from build123d import *

# Parameters (mm, degrees)
BOSS_EXTRUDE1_DEPTH = 11
SKETCH2_R           = 0.5
CUT_EXTRUDE1_DEPTH  = 39.49675311
SKETCH3_W           = 9
SKETCH3_H           = 20
BOSS_EXTRUDE2_DEPTH = 0.5
SKETCH5_R           = 1.25
SKETCH5_R_2         = 2
BOSS_EXTRUDE3_DEPTH = 0.5
FILLET2_R           = 0.5
FILLET3_R           = 0.5
FILLET4_R           = 0.5
FILLET5_R           = 0.5
FILLET6_R           = 0.5
FILLET7_R           = 0.5
CUT_EXTRUDE3_START  = -0.3
CUT_EXTRUDE3_DEPTH  = 0.3


with BuildPart() as part:
    # Sketch1 → Boss-Extrude1 (new body)
    with BuildSketch(Plane(origin=(0, 0, 0), x_dir=(0, 0, -1), z_dir=(1, 0, 0))):
        Polygon((0, 0), (0, 31), (20, 31), (20, 6), (14, 0), align=None)
    extrude(amount=BOSS_EXTRUDE1_DEPTH)

    # Sketch2 → Cut-Extrude1 (cut, through all)
    with BuildSketch(Plane(origin=(11, 0, 0), x_dir=(0, 0, -1), z_dir=(1, 0, 0))):
        with Locations((3, 2.8)):
            Circle(SKETCH2_R)
        with Locations((3, 28.2)):
            Circle(SKETCH2_R)
    extrude(amount=-CUT_EXTRUDE1_DEPTH, mode=Mode.SUBTRACT)

    # Sketch3 → Boss-Extrude2 (add)
    with BuildSketch(Plane.XY):
        with Locations((5.5, 18)):
            Rectangle(SKETCH3_W, SKETCH3_H)
    extrude(amount=BOSS_EXTRUDE2_DEPTH)

    # Sketch5 → Boss-Extrude3 (add)
    with BuildSketch(Plane(origin=(0, 31, 0), x_dir=(1, 0, 0), z_dir=(0, 1, 0))):
        with Locations(Location((3.5, 3.5, 0), (0, 0, 90))):
            Circle(SKETCH5_R)
        with Locations(Location((7.5, 3.5, 0), (0, 0, 90))):
            Circle(SKETCH5_R)
        with Locations(Location((5.5, 15, 0), (0, 0, 90))):
            Circle(SKETCH5_R_2)
        with Locations(Location((5.5, 9, 0), (0, 0, 90))):
            Circle(SKETCH5_R_2)
    extrude(amount=BOSS_EXTRUDE3_DEPTH)

    # Fillet2
    fillet2_edges = [part.edges().sort_by_distance(p)[0] for p in [
        (3.5, 31.5, -2.25),
    ]]
    fillet(fillet2_edges, radius=FILLET2_R - 0.0001)  # a hair under: the kernel refuses the full size

    # Fillet3
    fillet3_edges = [part.edges().sort_by_distance(p)[0] for p in [
        (7.5, 31.5, -2.25),
    ]]
    fillet(fillet3_edges, radius=FILLET3_R - 0.0001)  # a hair under: the kernel refuses the full size

    # Fillet4
    fillet4_edges = [part.edges().sort_by_distance(p)[0] for p in [
        (5.5, 31, 0),
    ]]
    fillet(fillet4_edges, radius=FILLET4_R)

    # Fillet5
    fillet5_edges = [part.edges().sort_by_distance(p)[0] for p in [
        (5.5, 31, -20),
    ]]
    fillet(fillet5_edges, radius=FILLET5_R)

    # Fillet6
    fillet6_edges = [part.edges().sort_by_distance(p)[0] for p in [
        (5.5, 0, 0),
    ]]
    fillet(fillet6_edges, radius=FILLET6_R)

    # Fillet7
    fillet7_edges = [part.edges().sort_by_distance(p)[0] for p in [
        (5.5, 6, -20),
    ]]
    fillet(fillet7_edges, radius=FILLET7_R)

    # Sketch6 → Cut-Extrude3 (cut)
    with BuildSketch(Plane(origin=(0, 31.5, 0), x_dir=(1, 0, 0), z_dir=(0, 1, 0)).offset(CUT_EXTRUDE3_START)):
        with BuildLine():
            Line((6.786176444, 10.531584197), (3.6331206, 8.282531321))
            ThreePointArc((3.6331206, 8.282531321), (3.86671689, 7.84570962), (4.200507105, 7.479697985))
            Line((4.200507105, 7.479697985), (7.373069331, 9.701149971))
            ThreePointArc((7.373069331, 9.701149971), (7.13328311, 10.15429038), (6.786176444, 10.531584197))
        make_face()
        with BuildLine():
            Line((3.62088338, 14.315222133), (6.812710383, 16.508904056))
            ThreePointArc((6.812710383, 16.508904056), (7.143293876, 16.139993525), (7.373069331, 15.701149971))
            Line((7.373069331, 15.701149971), (4.200507105, 13.479697985))
            ThreePointArc((4.200507105, 13.479697985), (3.856706124, 13.860006475), (3.62088338, 14.315222133))
        make_face()
    extrude(amount=CUT_EXTRUDE3_DEPTH, mode=Mode.SUBTRACT)


solid = part.part
For this review, take the finished solid that the model builds, in its own axes (mm). A direction names the side the tool comes from. Round coordinates to 2 decimals unless told otherwise and drop trailing zeros. Write each loop counter-clockwise with the first axis right and the second up, starting at its lowest first coordinate (ties: lowest second). Pieces come first, ordered by that corner, then holes. Notation, with made-up numbers: (72, 72.25) - (110, 72.25) arc R19 cw to (110, 103.25) - close; hole circle Ø2 at (-30, -30.75). An arc over 180 degrees is marked (long way). Use a Markdown table: item, result.
Q1. Clearance check with flat-ended pins moving along their axes: pin 1 (0.6 mm diameter, centred on x = 6.5, z = 0.5, fed in from -Y); pin 2 (0.6 mm diameter, centred on x = 4, z = 0.5, fed in from +Y); pin 3 (3.5 mm diameter, centred on x = 4, z = -13, fed in from +Y). State where each tip first meets the part, or that it passes through.
Derived:
| item | result |
|---|---|
| pin 1 | stops at y = 8 |
| pin 2 | stops at y = 28 |
| pin 3 | stops at y = 31.5 |
Q2. Wall thickness on line 1 along Y through (x, z) = (6, -3); line 2 along Y through (x, z) = (4.5, -3); line 3 along Y through (x, z) = (6.5, -7): over which ranges is each line inside the solid? List them lowest first.
Derived:
| item | result |
|---|---|
| line 1 | y = 0 to 2.3, 3.3 to 27.7, 28.7 to 31 |
| line 2 | y = 0 to 2.3, 3.3 to 27.7, 28.7 to 31.34 |
| line 3 | y = 0 to 31 |
Q3. The part is to be moulded in two halves that separate along Y. For faces 3 (the flat face through (5.23, 31.35, -9.42)), 4 (the cylindrical face through (5.6, 2.5, -2.6)), 5 (the flat face through (5, 0, -7)), 6 (the flat face through (3.5, 31.5, -3.5)), say which applies: pulls with the +Y half, pulls with the -Y half, needs draft (parallel to the pull), parting line crosses it, or undercut.
Derived:
| item | result |
|---|---|
| face 3 | needs draft |
| face 4 | undercut |
| face 5 | pulls with the -Y half |
| face 6 | pulls with the +Y half |
Q4. We need section B-B (z = -11.75). Give the boundary of the cut face in (x, y), plus the area to 3 significant figures.
Derived:
| item | result |
|---|---|
| outline | (0, 0) - (11, 0) - (11, 31) - (0, 31) - close |
| area | 341 mm2 |
Q5. We need section A-A (x = 1.75). Give the boundary of the cut face in (y, z), plus the area to 3 significant figures.
Derived:
| item | result |
|---|---|
| outline | (0, -14) - (5.85, -19.85) arc R0.5 ccw to (6.21, -20) - (30.5, -20) arc R0.5 ccw to (31, -19.5) - (31, -0.5) arc R0.5 ccw to (30.5, 0) - (28, 0) - (28, 0.5) - (8, 0.5) - (8, 0) - (0.5, 0) arc R0.5 ccw to (0, -0.5) - close; hole circle Ø1 at (2.8, -3); hole circle Ø1 at (28.2, -3) |
| area | 610 mm2 |
Q6. Machinability: for faces 1 (the cylindrical face through (3.814, 31.246, -16.075)), 2 (the cylindrical face through (5.577, 27.712, -2.892)), which of the approach directions +Z, -Z, +X, -X, +Y, -Y give a long, thin tool a straight path to every point of the face, cutting with its end or side? Answer none if there is none.
Derived:
| item | result |
|---|---|
| face 1 | +Y |
| face 2 | +X, -X |
